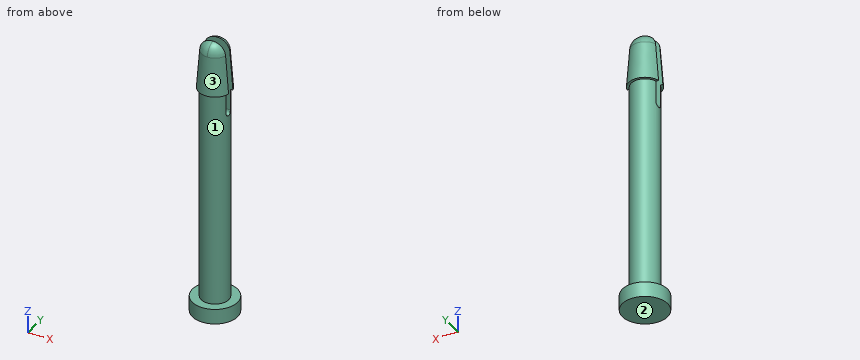
```python
from build123d import *

# Parameters (mm, degrees)
F0_R        = 4.5
F1_DEPTH    = 3
F2_R        = 2.75
F3_DEPTH    = 43
F6_W        = 10
F6_H        = 1.5
F7_DEPTH    = 15
F8_T2_ANGLE = 359.64
F8_T4_ANGLE = 359.64
F9_R        = 0.7499


# Not quite as in the source:
# - a fillet or chamfer that OpenCascade refuses, or shapes differently, is made with other operations: its cross-section is extruded or revolved along the edge and cut away or added
# - a fillet or chamfer is up to 0.001 mm smaller than in the source, because OpenCascade refuses the exact size


with BuildPart() as f1:
    # F0 (on Top) → F1 (new body)
    with BuildSketch(Plane.XY):
        Circle(F0_R)
    extrude(amount=F1_DEPTH)

    # F2 (on face) → F3 (join)
    with BuildSketch(Plane.XY.offset(3)):
        Circle(F2_R)
    extrude(amount=F3_DEPTH)

    # F4 (on Front) → F5 (revolve)
    with BuildSketch(Plane.XZ):
        Polygon((0, 56), (0, 46), (3.25, 46), (2.5, 56), align=None)
    revolve(axis=Axis((0, 0, 51), (0, 0, -1)))

    # F6 (on face) → F7 (cut)
    with BuildSketch(Plane.XY.offset(56)):
        Rectangle(F6_W, F6_H)
    extrude(amount=-F7_DEPTH, mode=Mode.SUBTRACT)

    # F8: fillet of radius 2.5 on 2 edges, made by hand

    # F8_s1 → F8_t2 (revolve, cut)
    with BuildSketch(Plane(origin=(0, 0, 0), x_dir=(0, 0, 1), z_dir=(0.9999950652, -0.0031415875, 0))):
        with BuildLine():
            ThreePointArc((56, 0.18047861), (55.3326807109, 1.880855454), (53.6869748706, 2.6734768847))
            Line((53.6869748706, 2.6734768847), (56, 2.5))
            Line((56, 2.5), (56, 0.18047861))
        make_face()
    revolve(axis=Axis((0, 0, 56), (0, 0, -1)), revolution_arc=F8_T2_ANGLE, mode=Mode.SUBTRACT)

    # F8_s3 → F8_t4 (revolve, cut)
    with BuildSketch(Plane(origin=(0, 0, 0), x_dir=(0, 0, 1), z_dir=(-0.9999950652, 0.0031415875, 0))):
        with BuildLine():
            ThreePointArc((53.6869748706, 2.6734768847), (55.3326807109, 1.880855454), (56, 0.18047861))
            Line((56, 0.18047861), (56, 2.5))
            Line((56, 2.5), (53.6869748706, 2.6734768847))
        make_face()
    revolve(axis=Axis((0, 0, 56), (0, 0, -1)), revolution_arc=F8_T4_ANGLE, mode=Mode.SUBTRACT)

    # F9 (radius 0.75 in the source; OpenCascade refuses exactly that, so slightly less here)
    f9_edges = [f1.edges().sort_by_distance(p)[0] for p in [
        (0, 0.75, 41),
        (0, -0.75, 41),
    ]]
    fillet(f9_edges, radius=F9_R)


solid = f1.part
```
Geometry check sheet. Reference: the model listing, model coordinates, mm. Face numbers are marked on the shaded views. Give positions to 0.01 mm unless a question says otherwise; leave off trailing zeros. Loops run counter-clockwise (first coordinate to the right, second up) from the corner with the lowest first, then second, coordinate; pieces in that order, holes last. Notation, with made-up numbers: M 63,89.5 L 121,89.5 A19 ccw 121,122.5 Z; hole C -25.75,51 d6. An arc over 180 degrees is marked long. Write item = value, one per line. Start each with the question number.
1. Thickness scan on probe 1 along Z at (x, y) = (-3.75, 0.5); probe 2 along Y at (x, z) = (0.75, 53.5); probe 3 along Y at (x, z) = (0, 53.5). Record the ranges inside material, lowest first.
2. Section check A-A, the plane z = 12.5. Enter the section's corners in (x, y).
3. Draft check along Z on the marked faces 1, 2 and 3. Enter one of: +Z half, -Z half, draft (parallel to the pull), parting line (faces both ways), or undercut.
4. Section check B-B, the plane z = 47. Enter the section's corners in (x, y) (3 decimals).
5. Section check C-C, the plane x = -3.75. Enter the section's corners in (y, z).
6. Go/stop test with flat-tipped pins: P1, Ø5, axis at x = -1, z = 33.5, coming from the -Y side; P2, Ø1.5, axis at x = 3, z = 50, coming from the +Y side; P3, Ø1.5, axis at x = -1, z = 14.5, coming from the +Y side. Record where each tip stops, or that it passes through.
Values follow:
q1.probe_1 = 0 to 3
q1.probe_2 = -2.58 to -0.75, 0.75 to 2.58
q1.probe_3 = -2.69 to -0.75, 0.75 to 2.69
q2.outline = C 0,0 d5.5
q3.face_1 = undercut
q3.face_2 = -Z half
q3.face_3 = +Z half
q4.outline = M -3.085,-0.75 A3.175 ccw 3.085,-0.75 Z; M -3.085,0.75 L 3.085,0.75 A3.175 ccw Z
q5.outline = M -2.49,0 L 2.49,0 L 2.49,3 L -2.49,3 Z
q6.P1 = -2.75
q6.P2 = 1.91
q6.P3 = 2.74
